For this review, use the dimensioned drawing (mm, ordinates from the lowest corner) and the shaded views. A direction names the side the tool comes from. Round coordinates to 2 decimals unless told otherwise and drop trailing zeros. Write each loop counter-clockwise with the first axis right and the second up, starting at its lowest first coordinate (ties: lowest second). Pieces come first, ordered by that corner, then holes. Notation, with made-up numbers: (65.25, -38) - (93.25, -38) arc R11 ccw to (93.25, -28) - close; hole circle Ø11 at (-0.75, 31.5). An arc over 180 degrees is marked (long way). Write each question's results on one line, items separated by ' | '.
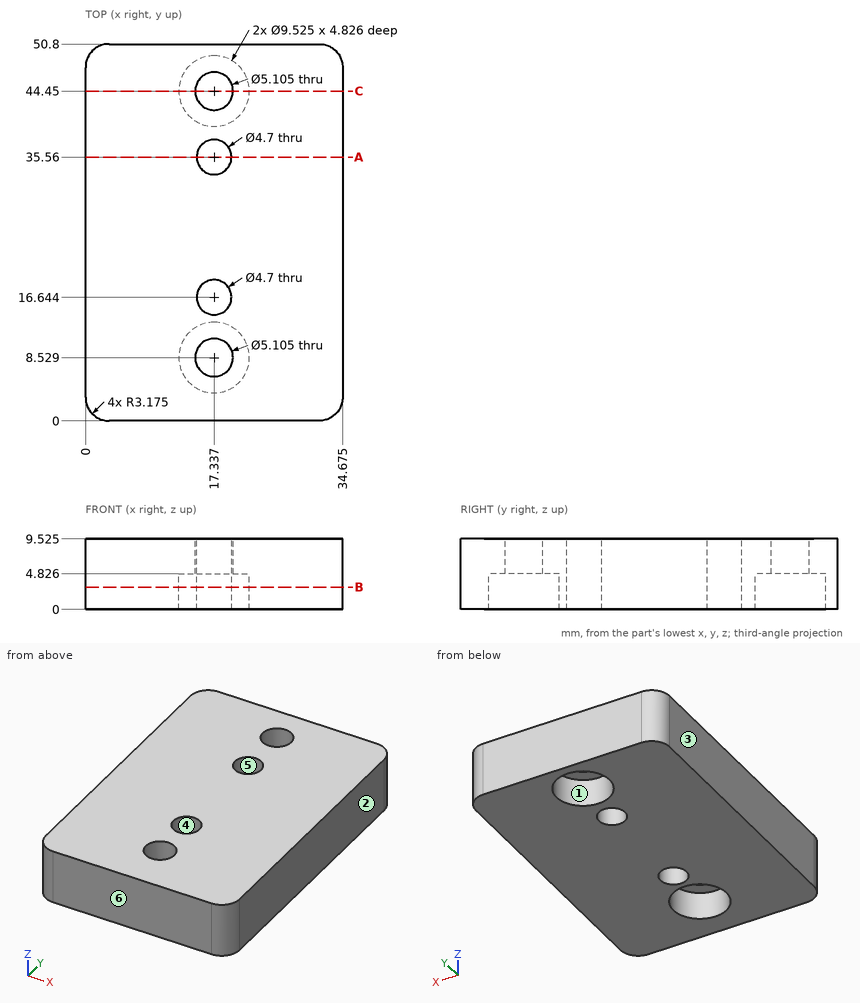
Q1. For probe 1 along Y at (x, z) = (19.5, 1.5) (1 decimal); probe 2 along Y at (x, z) = (18.5, 7.25) (1 decimal); probe 3 along Y at (x, z) = (13, 1.25) (1 decimal), list the stretches that pass through material, from the lowest coordinate up.
Evaluation:
probe 1: y = 0 to 4.3, 12.8 to 15.7, 17.6 to 34.6, 36.5 to 40.2, 48.7 to 50.8 | probe 2: y = 0 to 6.3, 10.8 to 14.6, 18.7 to 33.5, 37.6 to 42.2, 46.7 to 50.8 | probe 3: y = 0 to 6.6, 10.5 to 42.5, 46.4 to 50.8
Q2. We need section B-B (z = 3). State how many separate pieces and enclosed holes the cut face has, plus the area to 3 significant figures.
Evaluation:
separate pieces: 1 | enclosed holes: 4 | area: 1,580 mm^2
Q3. Insertion check: P1, Ø4.5, axis at x = 17.34, y = 44.45, coming from the +Z side; P2, Ø6.5, axis at x = 17.34, y = 8.53, coming from the -Z side. Each pin has a flat end and moves straight along its axis. Give the tip position at first contact, or say it passes through.
Evaluation:
P1: passes through | P2: stops at z = 4.83
Q4. The part is to be moulded in two halves that separate along X. For the marked faces 3, 4, 5 and 6, say which applies: released by +X, released by -X, zero draft, split by the parting line, or undercut.
Evaluation:
face 3: released by -X | face 4: undercut | face 5: undercut | face 6: zero draft
Q5. Tool access review of the marked faces 1 and 2: name each direction out of +Z, -Z, +X, -X, +Y, -Y from which nothing blocks a thin tool from reaching the whole face with its end or side.
Evaluation:
face 1: -Z | face 2: +Z, -Z, +X, +Y, -Y
Q6. We need section C-C (y = 44.45). State the section outline as (x, z) points (1 decimal).
Evaluation:
outline: (0, 0) - (12.6, 0) - (12.6, 4.8) - (14.8, 4.8) - (14.8, 9.5) - (0, 9.5) - close; (19.9, 4.8) - (22.1, 4.8) - (22.1, 0) - (34.7, 0) - (34.7, 9.5) - (19.9, 9.5) - close
Q7. We need section A-A (y = 35.56). State the section outline as (x, z) points (1 decimal).
Evaluation:
outline: (0, 0) - (15, 0) - (15, 9.5) - (0, 9.5) - close; (19.7, 0) - (34.7, 0) - (34.7, 9.5) - (19.7, 9.5) - close
